Geometry check sheet. Reference: the model listing, model coordinates, mm. Face numbers are marked on the shaded views. A direction names the side the tool comes from. Coordinates: 2 decimals unless noted, no trailing zeros. Write each loop counter-clockwise with the first axis right and the second up, starting at its lowest first coordinate (ties: lowest second). Pieces come first, ordered by that corner, then holes. Notation, with made-up numbers: M 76,71.25 L 127,71.25 A30 cw 127,94.25 Z; hole C -40,55 d9. An arc over 180 degrees is marked long. Put each result on its own line as item: value. Start each with the question number.
1) Scan lines: line 1 along X through (y, z) = (-0.25, 4.75); line 2 along Z through (x, y) = (16, 0.5); line 3 along Y through (x, z) = (3, 15). Record each from-to range of solid material in increasing order.
2) Cross-section at B-B on z = -3. Record the cut outline in (x, y), plus the area to 3 significant figures.
3) Gauge pin test, flat ends, axial feed: pin 1 (1.5 mm diameter, centred on y = 0, z = 9, fed in from +X); pin 2 (6 mm diameter, centred on y = 3.5, z = 9, fed in from -X); pin 3 (3 mm diameter, centred on y = 5, z = 17, fed in from +X); pin 4 (1 mm diameter, centred on y = 5.5, z = 17, fed in from -X). Record the tip position at first contact, or that the pin passes through.
4) Cross-section at A-A on x = -16. Record the cut outline in (y, z), plus the area to 3 significant figures.
5) Cross-section at C-C on y = -1.5. Record the cut outline in (x, z).
6) Set-up check for the marked faces 1, 2, 3 and 4: record each of +Z, -Z, +X, -X, +Y, -Y from which the full face is reachable in a straight line by a thin tool's end or side.
7) Mould release check, pull along X, two halves, no side actions. Record for the marked faces 5, 6 and 7: released by +X, released by -X, zero draft, split by the parting line, or undercut.
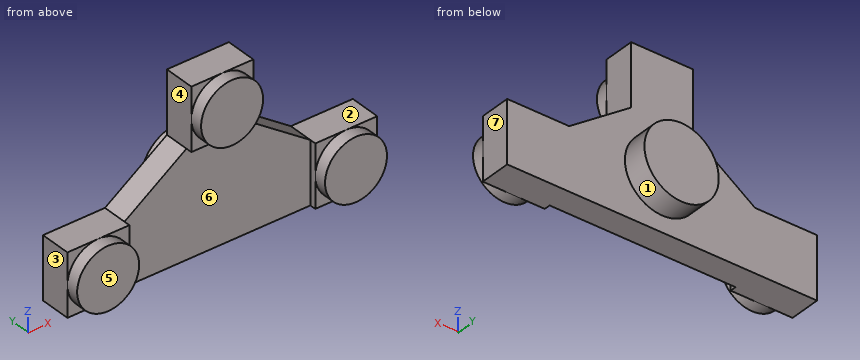
from build123d import *

# Parameters (mm, degrees)
EXTRUDE_1_DEPTH = 4
SKETCH_1_W      = 10
SKETCH_1_H      = 10
EXTRUDE_2_DEPTH = 1
SKETCH_5_R      = 6
EXTRUDE_3_DEPTH = 4
SKETCH_6_R      = 5
EXTRUDE_4_DEPTH = 2


with BuildPart() as part:
    # 草图2 → 凸台-拉伸1 (new body)
    with BuildSketch(Plane(origin=(0, 0, 0), x_dir=(1, 0, 0), z_dir=(0, 1, 0))):
        Polygon((-5, -22), (5, -22), (5, -12), (15, -5), (25, -5), (25, 5), (-25, 5), (-25, -5), (-15, -5), (-5, -12), align=None)
    extrude(amount=EXTRUDE_1_DEPTH)

    # 草图1 → 凸台-拉伸2 (add)
    with BuildSketch(Plane(origin=(0, 0, 0), x_dir=(1, 0, 0), z_dir=(0, 1, 0))):
        with Locations((-20, 0)):
            Rectangle(SKETCH_1_W, SKETCH_1_H)
        with Locations((20, 0)):
            Rectangle(SKETCH_1_W, SKETCH_1_H)
        with Locations((0, -17)):
            Rectangle(SKETCH_1_W, SKETCH_1_H)
    extrude(amount=-EXTRUDE_2_DEPTH)

    # 草图5 → 凸台-拉伸3 (add)
    with BuildSketch(Plane(origin=(0, 4, 0), x_dir=(1, 0, 0), z_dir=(0, 1, 0))):
        with Locations((0, -3.6)):
            Circle(SKETCH_5_R)
    extrude(amount=EXTRUDE_3_DEPTH)

    # 草图6 → 凸台-拉伸4 (add)
    with BuildSketch(Plane.XZ.offset(1)):
        with Locations((0, 17)):
            Circle(SKETCH_6_R)
        with Locations((20, 0)):
            Circle(SKETCH_6_R)
        with Locations((-20, 0)):
            Circle(SKETCH_6_R)
    extrude(amount=EXTRUDE_4_DEPTH)


solid = part.part
Answer key:
1. line 1: x = -25 to -15, 15 to 25
1. line 2: z = -5 to 5
1. line 3: y = -3 to 4
2. outline: M -25,-1 L -24,-1 L -24,-3 L -16,-3 L -16,-1 L -15,-1 L -15,0 L 15,0 L 15,-1 L 16,-1 L 16,-3 L 24,-3 L 24,-1 L 25,-1 L 25,4 L -25,4 Z
2. area: 252 mm²
3. pin 1: stops at x = 10.36
3. pin 2: stops at x = -13.57
3. pin 3: stops at x = 5
3. pin 4: passes through
4. outline: M -3,-3 L -1,-3 L -1,-5 L 4,-5 L 4,5 L -1,5 L -1,3 L -3,3 Z
4. area: 62.0 mm²
5. outline: C -20,0 d10; C 0,17 d10; C 20,0 d10
6. face 1: +Y
6. face 2: +Z, +X, +Y, -Y
6. face 3: +Z, -Z, -X, +Y, -Y
6. face 4: +Z, -X, +Y, -Y
7. face 5: zero draft
7. face 6: undercut
7. face 7: released by +X
